Answer from the drawing. Dimensions are ordinates in mm from the lowest x, y and z of the part. A direction names the side the tool comes from. Round coordinates to 2 decimals unless told otherwise and drop trailing zeros. Write each loop counter-clockwise with the first axis right and the second up, starting at its lowest first coordinate (ties: lowest second). Pieces come first, ordered by that corner, then holes.
1. Straight lines are drawn through the part: probe 1 along Z at (x, y) = (947, 384); probe 2 along Y at (x, z) = (1177, 620.5); probe 3 along X at (y, z) = (139.5, 794). For each, find the intervals that lie inside material, in ascending order.
2. A tool of negligible diameter and unlimited length cuts with its end or side. For the marked faces 1, 2 and 3, from which of +Z, -Z, +X, -X, +Y, -Y can it reach the whole face along a straight path? Write none if from no direction.
3. Find section B-B (x = 500). Write down the section's boundary in (y, z).
4. Find section A-A (z = 450). Write down the section's boundary in (x, y).
5. Find section C-C (y = 64). Write down the section's boundary in (x, z).
6. Find section D-D (x = 1297). Write down the section's boundary in (y, z).
7. Flat-ended cylindrical pins translate along their axes: pin 1 Ø6 at (x, y) = (558.5, 455) entering from +Z; pin 2 Ø1.5 at (y, z) = (333.5, 392.5) entering from -X; pin 3 Ø12 at (x, y) = (534.5, 394.5) entering from -Z; pin 4 Ø1.5 at (x, y) = (549.5, 116.5) entering from +Z. Find the tip coordinate at first contact, or state that the pin passes through.
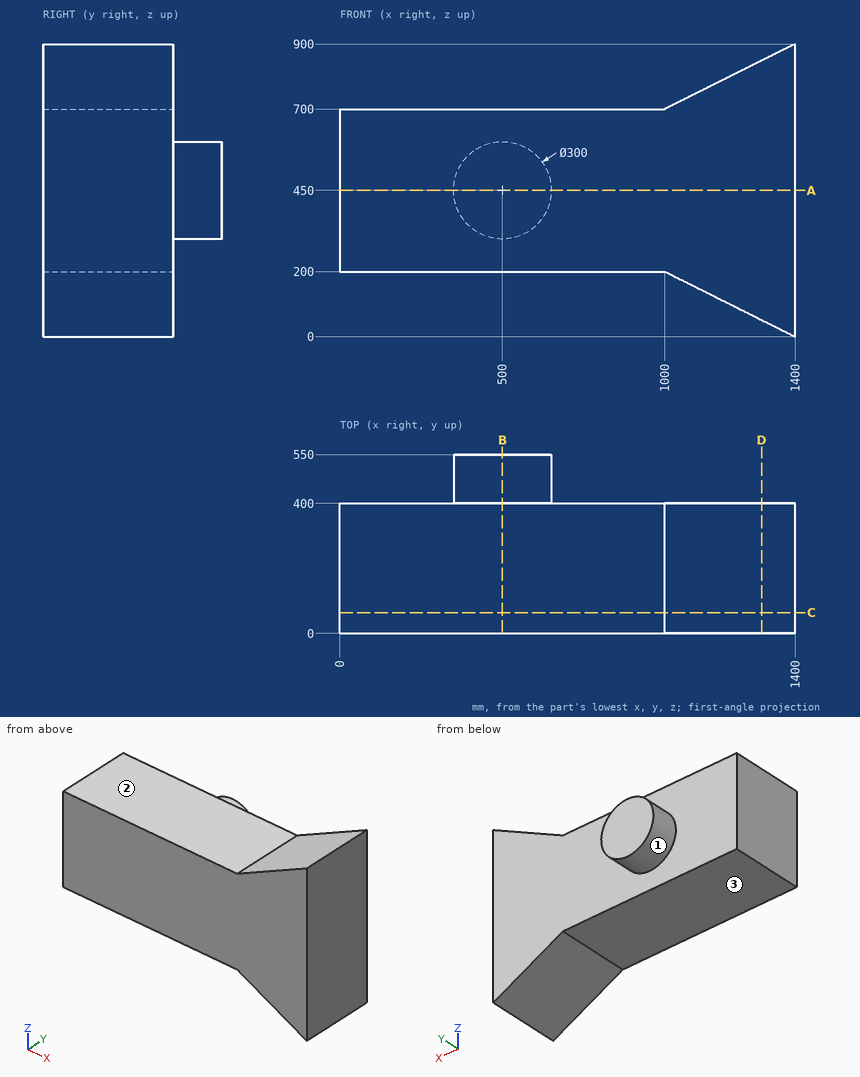
Worked answers:
1. probe 1: z = 200 to 700
1. probe 2: y = 0 to 400
1. probe 3: x = 1188 to 1400
2. face 1: +Y
2. face 2: +Z, -X, +Y, -Y
2. face 3: -Z, -X, +Y, -Y
3. outline: (0, 200) - (400, 200) - (400, 300) - (550, 300) - (550, 600) - (400, 600) - (400, 700) - (0, 700) - close
4. outline: (0, 0) - (1400, 0) - (1400, 400) - (650, 400) - (650, 550) - (350, 550) - (350, 400) - (0, 400) - close
5. outline: (0, 200) - (1000, 200) - (1400, 0) - (1400, 900) - (1000, 700) - (0, 700) - close
6. outline: (0, 51.5) - (400, 51.5) - (400, 848.5) - (0, 848.5) - close
7. pin 1: stops at z = 589.35
7. pin 2: stops at x = 0
7. pin 3: stops at z = 200
7. pin 4: stops at z = 700
